For this review, take the finished solid that the model builds, in its own axes (mm). Coordinates: 2 decimals unless noted, no trailing zeros. Loops run counter-clockwise (first coordinate to the right, second up) from the corner with the lowest first, then second, coordinate; pieces in that order, holes last. Notation, with made-up numbers: (-36.5, 63) -> (-25.5, 63) arc R17 ccw to (-25.5, 79) -> close; hole circle Ø2 at (-25.75, 35). An arc over 180 degrees is marked (long way). One line per item, written item: value.
from build123d import *

# Parameters (mm, degrees)
SKETCH1_W               = 76.2
SKETCH1_H               = 63.5
BOSS_EXTRUDE1_DEPTH     = 1.5875
F_3_8_CLEARANCE_HOLE1_D = 9.8044
F_1_2_CLEARANCE_HOLE1_D = 13.09624
CHAMFER1_SIZE           = 25.4
CHAMFER2_SIZE           = 6.35


with BuildPart() as part:
    # Sketch1 → Boss-Extrude1 (new, symmetric)
    with BuildSketch(Plane(origin=(0, 0, 0), x_dir=(1, 0, 0), z_dir=(0, 1, 0))):
        Rectangle(SKETCH1_W, SKETCH1_H)
    extrude(amount=BOSS_EXTRUDE1_DEPTH, both=True)

    # 3/8 Clearance Hole1 (through all)
    with Locations(Plane(origin=(0, 1.5875, 0), x_dir=(1, 0, 0), z_dir=(0, 1, 0))):
        with Locations((0, 19.05), (25.4, 19.05), (-25.4, 19.05)):
            Hole(F_3_8_CLEARANCE_HOLE1_D / 2)

    # 1/2 Clearance Hole1 (through all)
    with Locations(Plane(origin=(0, 1.5875, 0), x_dir=(1, 0, 0), z_dir=(0, 1, 0))):
        with Locations((0, -12.7)):
            Hole(F_1_2_CLEARANCE_HOLE1_D / 2)

    # Chamfer1
    chamfer1_edges = [part.edges().sort_by_distance(p)[0] for p in [
        (38.1, 0, 31.75),
        (-38.1, 0, 31.75),
    ]]
    chamfer(chamfer1_edges, length=CHAMFER1_SIZE)

    # Chamfer2
    chamfer2_edges = [part.edges().sort_by_distance(p)[0] for p in [
        (-38.1, 0, -31.75),
        (38.1, 0, -31.75),
    ]]
    chamfer(chamfer2_edges, length=CHAMFER2_SIZE)


solid = part.part
1. Take a section at C-C, the plane z = -19.05. Give the boundary of the cut face in (x, y).
Return value:
outline: (-38.1, -1.59) -> (-30.3, -1.59) -> (-30.3, 1.59) -> (-38.1, 1.59) -> close; (-20.5, -1.59) -> (-4.9, -1.59) -> (-4.9, 1.59) -> (-20.5, 1.59) -> close; (4.9, -1.59) -> (20.5, -1.59) -> (20.5, 1.59) -> (4.9, 1.59) -> close; (30.3, -1.59) -> (38.1, -1.59) -> (38.1, 1.59) -> (30.3, 1.59) -> close
2. Insertion check: pin 1 Ø9 at (x, z) = (25.4, -19.05) entering from +Y. The pin has a flat end and moves straight along its axis. Give the tip position at first contact, or say it passes through.
Return value:
pin 1: passes through
3. Take a section at B-B, the plane x = 25.4. Give the boundary of the cut face in (y, z).
Return value:
outline: (-1.59, -31.75) -> (1.59, -31.75) -> (1.59, -23.95) -> (-1.59, -23.95) -> close; (-1.59, -14.15) -> (1.59, -14.15) -> (1.59, 19.05) -> (-1.59, 19.05) -> close
4. To check wall thickness, follow probe 1 along Z at (x, y) = (0, -0.8); probe 2 along X at (y, z) = (-0.65, -19.05); probe 3 along Z at (x, y) = (3.5, -1.4). State the ranges of each line that lie inside material, in increasing order. Write a range as from..to.
Return value:
probe 1: z = -31.75..-23.95, -14.15..6.15, 19.25..31.75
probe 2: x = -38.1..-30.3, -20.5..-4.9, 4.9..20.5, 30.3..38.1
probe 3: z = -31.75..-22.48, -15.62..7.17, 18.23..31.75
5. The part is to be moulded in two halves that separate along Z. For faces 1 (the flat face through (25.58, -0.02, 18.87)), 2 (the cylindrical face through (0.64, -0.02, -23.91)), 3 (the flat face through (-1, -1.588, 0)), say which applies: pulls with the +Z half, pulls with the -Z half, needs draft (parallel to the pull), parting line crosses it, or undercut.
Return value:
face 1: pulls with the +Z half
face 2: undercut
face 3: needs draft
6. Take a section at D-D, the plane y = 0. Give the boundary of the cut face in (x, z).
Return value:
outline: (-38.1, -25.4) -> (-31.75, -31.75) -> (31.75, -31.75) -> (38.1, -25.4) -> (38.1, 6.35) -> (12.7, 31.75) -> (-12.7, 31.75) -> (-38.1, 6.35) -> close; hole circle Ø9.8 at (-25.4, -19.05); hole circle Ø13.1 at (0, 12.7); hole circle Ø9.8 at (0, -19.05); hole circle Ø9.8 at (25.4, -19.05)
7. Take a section at A-A, the plane z = 12.7. Give the boundary of the cut face in (x, y).
Return value:
outline: (-31.75, -1.59) -> (-6.55, -1.59) -> (-6.55, 1.59) -> (-31.75, 1.59) -> close; (6.55, -1.59) -> (31.75, -1.59) -> (31.75, 1.59) -> (6.55, 1.59) -> close
